Part model, mm, in its own coordinate system. A direction names the side the tool comes from. Round coordinates to 2 decimals unless told otherwise and drop trailing zeros. Loops run counter-clockwise (first coordinate to the right, second up) from the corner with the lowest first, then second, coordinate; pieces in that order, holes last. Notation, with made-up numbers: (-11, 13) - (-6, 13) arc R24 cw to (-6, 37) - close; hole circle Ø10 at (10, 49). An arc over 180 degrees is marked (long way). Put each result on its own line as item: value.
from build123d import *

# Parameters (mm, degrees)
CORTAR_EXTRUIR1_DEPTH = 5
REDONDEO1_R           = 1
REDONDEO2_R           = 0.5
CHAFL_N1_SIZE         = 0.5


with BuildPart() as part:
    # Croquis1 → Revolución1 (revolve)
    with BuildSketch(Plane.XY, mode=Mode.PRIVATE) as revoluci_n1_sk:
        Polygon((0, 0), (0, 8), (10, 8), (10, 5), (35, 5), (35, 0), align=None)
    revolve(revoluci_n1_sk.sketch.rotate(Axis((0, 0, 0), (1, 0, 0)), 90), axis=Axis((0, 0, 0), (1, 0, 0)))

    # Croquis2 → Cortar-Extruir1 (cut)
    with BuildSketch(Plane.ZY):
        Polygon((0, 4.618802154), (-4, 2.309401077), (-4, -2.309401077), (0, -4.618802154), (4, -2.309401077), (4, 2.309401077), align=None)
    extrude(amount=-CORTAR_EXTRUIR1_DEPTH, mode=Mode.SUBTRACT)

    # Redondeo1
    redondeo1_edges = [part.edges().sort_by_distance(p)[0] for p in [
        (0, 0, -8),
    ]]
    fillet(redondeo1_edges, radius=REDONDEO1_R)

    # Redondeo2
    redondeo2_edges = [part.edges().sort_by_distance(p)[0] for p in [
        (10, 0, -5),
    ]]
    fillet(redondeo2_edges, radius=REDONDEO2_R)

    # Chaflán1
    chafl_n1_edges = [part.edges().sort_by_distance(p)[0] for p in [
        (35, 0, -5),
    ]]
    chamfer(chafl_n1_edges, length=CHAFL_N1_SIZE)


solid = part.part
1. Two-plate mould, pull along Z, no slides. Class faces 1 (the flat face through (10, -5.4, 1.7)), 2 (the cylindrical face through (5.56, 7.81, -1.73)), 3 (the flat face through (2.46, -3.48, 1.97)): pulls with the +Z half, pulls with the -Z half, needs draft (parallel to the pull), parting line crosses it, or undercut.
A:
face 1: needs draft
face 2: parting line crosses it
face 3: undercut
2. Band-saw the part on A-A (y = 0). List the corners of the cut face in (x, z).
A:
outline: (0, -7) arc R1 ccw to (1, -8) - (10, -8) - (10, -5.5) arc R0.5 cw to (10.5, -5) - (34.5, -5) - (35, -4.5) - (35, 4.5) - (34.5, 5) - (10.5, 5) arc R0.5 cw to (10, 5.5) - (10, 8) - (1, 8) arc R1 ccw to (0, 7) - (0, 4) - (5, 4) - (5, -4) - (0, -4) - close
3. Probe line 1 along Z through (x, y) = (2, 0.25); line 2 along Y through (x, z) = (28, -0.25); line 3 along X through (y, z) = (-0.25, -6.75). List the from-to ranges inside material, lowest first. Write a range as [from, to].
A:
line 1: z = [-8, -4], [4, 8]
line 2: y = [-4.99, 4.99]
line 3: x = [0, 10]
4. Tool access for faces 4 (the flat face through (2.46, 3.48, -1.97)), 5 (the cylindrical face through (23, 0, -5)), 6 (the flat face through (0, 5, 0)): list every direction of +Z, -Z, +X, -X, +Y, -Y with a clear straight run to the whole face (end or side of a thin tool).
A:
face 4: -X
face 5: +X
face 6: +Z, -Z, -X, +Y, -Y
5. Pin check, flat tips, straight feed: P1, Ø2, axis at x = 27.5, z = 2, coming from the +Y side; P2, Ø3, axis at x = 17.5, z = -5, coming from the +Y side; P3, Ø5, axis at x = 31.5, y = 0, coming from the -Z side. Stop position of each tip, or through.
A:
P1: stops at y = 4.9
P2: stops at y = 3.57
P3: stops at z = -5
6. Band-saw the part on B-B (x = 20.5). List the corners of the cut face in (y, z), plus the area to 3 significant figures.
A:
outline: circle Ø10 at (0, 0)
area: 78.5 mm²
